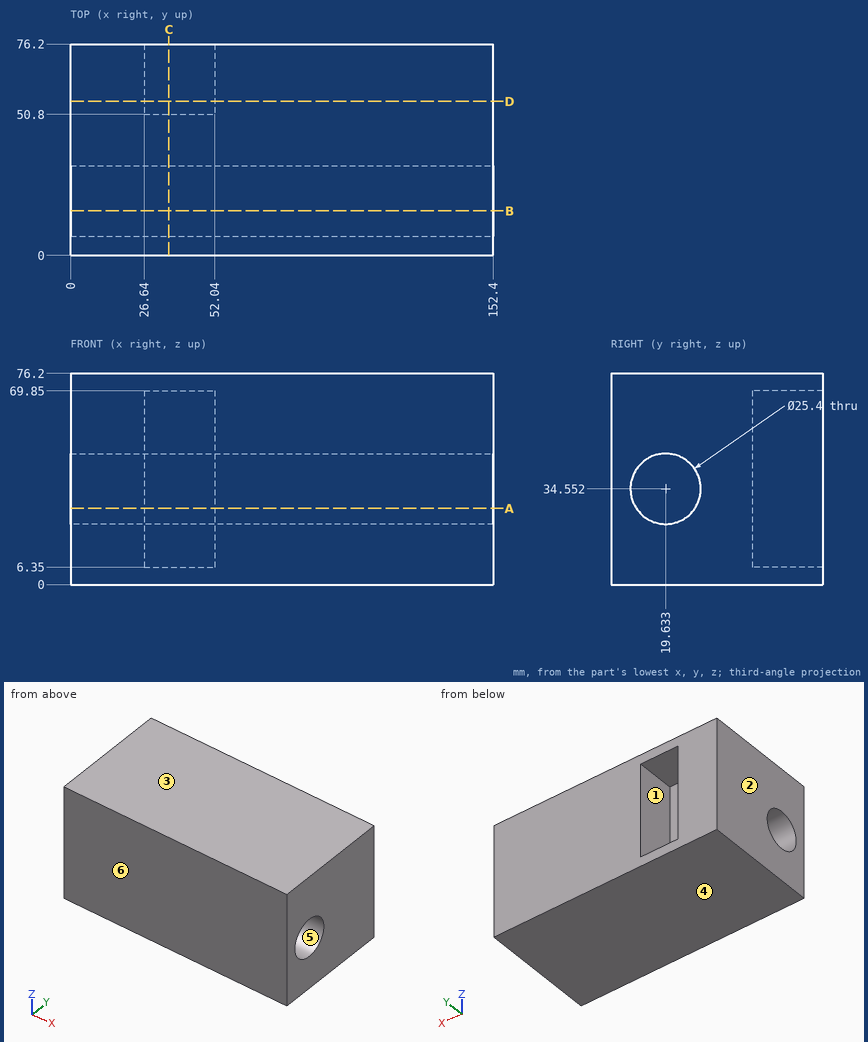
Design review of the part shown in the three views and the two pictorial views. Dimensions are in mm from the part's minimum x, y and z. A direction names the side the tool comes from. Round coordinates to 2 decimals unless told otherwise and drop trailing zeros. Write each loop counter-clockwise with the first axis right and the second up, starting at its lowest first coordinate (ties: lowest second). Pieces come first, ordered by that corner, then holes.
Item 1: For the marked faces 1 and 2, list the 3-axis set-ups (+Z, -Z, +X, -X, +Y, -Y) from which the entire face can be reached by the end or side of a thin tool; tool diameter is ignored.
Item 2: We need section B-B on y = 16. Write out the cut boundary in (x, z).
Item 3: We need section C-C on x = 35.5. Write out the cut boundary in (y, z).
Item 4: Clearance check with flat-ended pins moving along their axes: pin 1 Ø20.5 at (y, z) = (19.63, 34.55) entering from +X; pin 2 Ø12.5 at (x, z) = (36.5, 34.5) entering from +Y. State where each tip first meets the part, or that it passes through.
Item 5: The part is to be moulded in two halves that separate along Z. For the marked faces 3, 4, 5 and 6, say which applies: +Z half, -Z half, draft (parallel to the pull), parting line (faces both ways), or undercut.
Item 6: We need section D-D on y = 55.5. Write out the cut boundary in (x, z), and give its area (4 significant figures).
Item 7: We need section A-A on z = 27.5. Write out the cut boundary in (x, y) (1 decimal), and give its area (3 significant figures).
Item 8: For probe 1 along X at (y, z) = (54, 15); probe 2 along Y at (x, z) = (37.5, 56.5); probe 3 along Z at (x, y) = (134.5, 23), list the stretches that pass through material, from the lowest coordinate up.
Returned:
1. face 1: +Y
1. face 2: +Z, -Z, -X, +Y, -Y
2. outline: (0, 0) - (152.4, 0) - (152.4, 22.38) - (0, 22.38) - close; (0, 46.72) - (152.4, 46.72) - (152.4, 76.2) - (0, 76.2) - close
3. outline: (0, 0) - (76.2, 0) - (76.2, 6.35) - (50.8, 6.35) - (50.8, 69.85) - (76.2, 69.85) - (76.2, 76.2) - (0, 76.2) - close; hole circle Ø25.4 at (19.63, 34.55)
4. pin 1: passes through
4. pin 2: stops at y = 50.8
5. face 3: +Z half
5. face 4: -Z half
5. face 5: undercut
5. face 6: draft
6. outline: (0, 0) - (152.4, 0) - (152.4, 76.2) - (0, 76.2) - close; hole (26.64, 6.35) - (52.04, 6.35) - (52.04, 69.85) - (26.64, 69.85) - close
6. area: 10,000 mm2
7. outline: (0, 0) - (152.4, 0) - (152.4, 9.1) - (0, 9.1) - close; (0, 30.2) - (152.4, 30.2) - (152.4, 76.2) - (52, 76.2) - (52, 50.8) - (26.6, 50.8) - (26.6, 76.2) - (0, 76.2) - close
7. area: 7,750 mm2
8. probe 1: x = 0 to 26.64, 52.04 to 152.4
8. probe 2: y = 0 to 50.8
8. probe 3: z = 0 to 22.31, 46.8 to 76.2
